from build123d import *

# Parameters (mm, degrees)
SKETCH_1_W          = 123
SKETCH_1_H          = 120
SKETCH_1_R          = 2
EXTRUDE_1_DEPTH     = 30
SKETCH_2_W          = 15
SKETCH_2_H          = 54
CUT_EXTRUDE_1_DEPTH = 120


with BuildPart() as part:
    # 草图1 → 凸台-拉伸1 (new body)
    with BuildSketch(Plane.XY):
        with Locations((-25.906926203, 53.207805922)):
            Rectangle(SKETCH_1_W, SKETCH_1_H)
        with Locations((-84.008388051, 109.894431899)):
            Circle(SKETCH_1_R, mode=Mode.SUBTRACT)
        with Locations(Location((32.194535644, 109.894431899, 0), (0, 0, 180))):
            Circle(SKETCH_1_R, mode=Mode.SUBTRACT)
        with Locations((32.194535644, -3.478820055)):
            Circle(SKETCH_1_R, mode=Mode.SUBTRACT)
        with Locations(Location((-84.008388051, -3.478820055, 0), (0, 0, 180))):
            Circle(SKETCH_1_R, mode=Mode.SUBTRACT)
        with BuildLine():
            Line((-72.406926203, 111.207805922), (20.593073797, 111.207805922))
            ThreePointArc((20.593073797, 111.207805922), (29.785461952, 107.400194077), (33.593073797, 98.207805922))
            Line((33.593073797, 98.207805922), (33.593073797, 8.207805922))
            ThreePointArc((33.593073797, 8.207805922), (29.785461952, -0.984582233), (20.593073797, -4.792194078))
            Line((20.593073797, -4.792194078), (-72.406926203, -4.792194078))
            ThreePointArc((-72.406926203, -4.792194078), (-81.599314359, -0.984582233), (-85.406926203, 8.207805922))
            Line((-85.406926203, 8.207805922), (-85.406926203, 98.207805922))
            ThreePointArc((-85.406926203, 98.207805922), (-81.599314359, 107.400194077), (-72.406926203, 111.207805922))
        make_face(mode=Mode.SUBTRACT)
    extrude(amount=EXTRUDE_1_DEPTH)

    # 草图2 → 切除-拉伸1 (cut)
    with BuildSketch(Plane(origin=(35.593073797, 0, 0), x_dir=(0, 0, -1), z_dir=(1, 0, 0))):
        with Locations((-10.186283232, 79.999305489)):
            Rectangle(SKETCH_2_W, SKETCH_2_H)
    extrude(amount=-CUT_EXTRUDE_1_DEPTH, mode=Mode.SUBTRACT)


solid = part.part
Check sheet for the modelled part. Datum: model origin and axes. Units: mm. A direction names the side the tool comes from. Give positions to 0.01 mm unless a question says otherwise; leave off trailing zeros. Order: outer loops, then holes, each group sorted by start corner. A loop starts at its lowest first (then second) coordinate and runs counter-clockwise, first axis right, second up. Notation, with made-up numbers: (89.5, -10) - (124.5, -10) arc R21 cw to (124.5, 0) - close; hole circle Ø3 at (66.25, 70). An arc over 180 degrees is marked (long way). Answer as CSV lines item,"result".
1. Mould release check, pull along Y, two halves, no side actions. Record for faces 4 (the face through (30.196, -3.391, 14.79)), 5 (the face through (-87.407, 52, 15)), 6 (the face through (-27, -6.792, 15)): released by +Y, released by -Y, zero draft, split by the parting line, or undercut.
Result sheet:
face 4,"undercut"
face 5,"zero draft"
face 6,"released by -Y"
2. Go/stop test with flat-tipped pins: P1, Ø4.5, axis at x = 32.5, y = 70.5, coming from the -Z side; P2, Ø1.1, axis at y = 105, z = 13, coming from the +X side. Record where each tip stops, or that it passes through.
Result sheet:
P1,"z = 0"
P2,"x = -84.41"
3. Section check A-A (x = -60). Record the boundary of the cut face in (y, z), then the cut area to 3 significant figures.
Result sheet:
outline,"(-6.79, 0) - (-4.79, 0) - (-4.79, 30) - (-6.79, 30) - close; (111.21, 0) - (113.21, 0) - (113.21, 30) - (111.21, 30) - close"
area,"120 mm²"
4. Section check C-C (y = 92). Record the boundary of the cut face in (x, z), then the cut area to 3 significant figures.
Result sheet:
outline,"(-87.41, 0) - (-85.41, 0) - (-85.41, 30) - (-87.41, 30) - close; (33.59, 0) - (35.59, 0) - (35.59, 2.69) - (33.59, 2.69) - close; (33.59, 17.69) - (35.59, 17.69) - (35.59, 30) - (33.59, 30) - close"
area,"90.0 mm²"
5. Scan lines: probe 1 along X at (y, z) = (66.5, 19); probe 2 along Y at (x, z) = (-60, 22); probe 3 along Y at (x, z) = (25, 8.5). Record each from-to range of solid material in increasing order. Write a range as from..to.
Result sheet:
probe 1,"-87.41..-85.41, 33.59..35.59"
probe 2,"-6.79..-4.79, 111.21..113.21"
probe 3,"-6.79..-4.02, 110.44..113.21"
6. Section check D-D (z = 11.5). Record the boundary of the cut face in (x, y), then the cut area to 3 significant figures.
Result sheet:
outline,"(-87.41, -6.79) - (35.59, -6.79) - (35.59, 53) - (33.59, 53) - (33.59, 8.21) arc R13 cw to (20.59, -4.79) - (-72.41, -4.79) arc R13 cw to (-85.41, 8.21) - (-85.41, 98.21) arc R13 cw to (-84.41, 103.21) - (-84.41, 107) - (-81.98, 107) arc R13 cw to (-72.41, 111.21) - (20.59, 111.21) arc R13 cw to (30.17, 107) - (35.59, 107) - (35.59, 113.21) - (-87.41, 113.21) - close; hole circle Ø4 at (-84.01, -3.48); hole circle Ø4 at (-84.01, 109.89); hole circle Ø4 at (32.19, -3.48); hole circle Ø4 at (32.19, 109.89)"
area,"929 mm²"
7. Section check B-B (y = 36.5). Record the boundary of the cut face in (x, z), then the cut area to 3 significant figures.
Result sheet:
outline,"(-87.41, 0) - (-85.41, 0) - (-85.41, 30) - (-87.41, 30) - close; (33.59, 0) - (35.59, 0) - (35.59, 30) - (33.59, 30) - close"
area,"120 mm²"
8. Tool access check on faces 1 (the face through (-27, 113.208, 15)), 2 (the face through (33, 106.999, 10)), 3 (the face through (-81.7, 107.3, 14.8)). Record the directions out of +Z, -Z, +X, -X, +Y, -Y that give a thin tool (end or side, any length) a straight path to the whole face; none if there is none.
Result sheet:
face 1,"+Z, -Z, +X, -X, +Y"
face 2,"+X"
face 3,"+Z, -Z"
